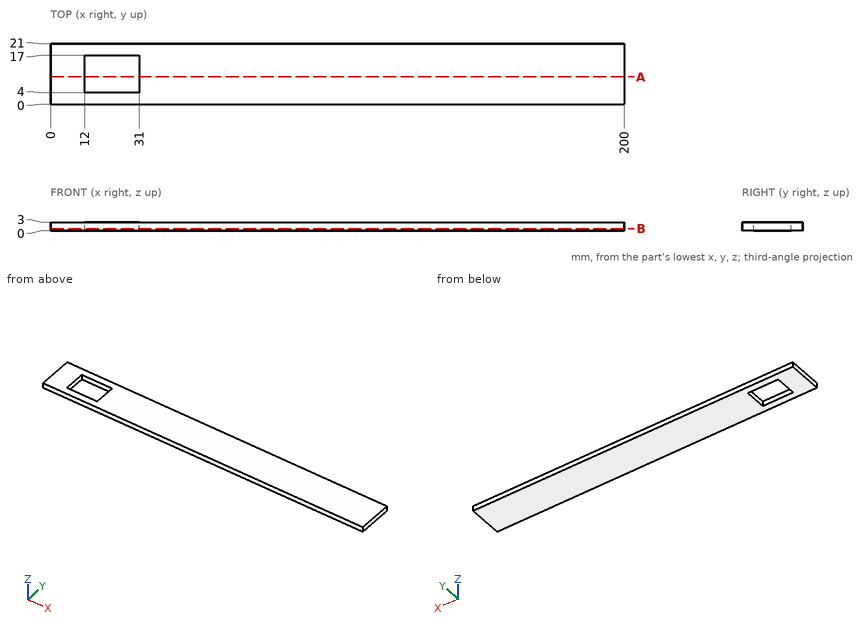
Answer from the drawing. Dimensions are ordinates in mm from the lowest x, y and z of the part. Give positions to 0.01 mm unless a question says otherwise; leave off trailing zeros. Order: outer loops, then holes, each group sorted by start corner. A loop starts at its lowest first (then second) coordinate and runs counter-clockwise, first axis right, second up. Notation, with made-up numbers: (62, 27) - (70, 27) arc R17 cw to (70, 59) - close; hole circle Ø6 at (-6.5, 42). An arc over 180 degrees is marked (long way). One line per item, written item: value. Start each with the question number.
1. Section A-A, the plane y = 9.5 is taken. Write down the section's boundary in (x, z), then the cut area to 3 significant figures.
2. Section B-B, the plane z = 0.8 is taken. Write down the section's boundary in (x, y).
3. Consider line 1 (X direction, y = 8.5, z = 0.35); line 2 (Y direction, x = 17.5, z = 1.3). Determine where each line is inside the solid, lowest interval first.
Filled sheet:
1. outline: (0, 0) - (12, 0) - (12, 3) - (0, 3) - close; (31, 0) - (200, 0) - (200, 3) - (31, 3) - close
1. area: 543 mm²
2. outline: (0, 0) - (200, 0) - (200, 21) - (0, 21) - close; hole (12, 4) - (31, 4) - (31, 17) - (12, 17) - close
3. line 1: 0 to 12, 31 to 200
3. line 2: 0 to 4, 17 to 21
